```python
from build123d import *

# Parameters (mm, degrees)
SKETCH1_W           = 30
SKETCH1_H           = 80
BOSS_EXTRUDE1_DEPTH = 5
SKETCH2_W           = 5
SKETCH2_H           = 26.5
SKETCH2_H_2         = 5
SKETCH2_R           = 1.5
CUT_EXTRUDE1_DEPTH  = 5
BOSS_EXTRUDE2_DEPTH = 5
FILLET1_R           = 30
SKETCH5_R           = 6.55
SKETCH5_R_2         = 1.5
CUT_EXTRUDE2_DEPTH  = 5
SKETCH6_W           = 16.25
SKETCH6_H           = 5
SKETCH6_R           = 1.5
CUT_EXTRUDE3_DEPTH  = 10
SKETCH7_W           = 5
SKETCH7_H           = 5.5
SKETCH7_H_2         = 10
SKETCH7_H_3         = 6
SKETCH7_R           = 1.5
CUT_EXTRUDE4_DEPTH  = 10
SKETCH8_W           = 5.078430198
SKETCH8_H           = 27.315407993
SKETCH8_W_2         = 5
SKETCH8_H_2         = 26.5
BOSS_EXTRUDE4_DEPTH = 5


with BuildPart() as part:
    # Sketch1 → Boss-Extrude1 (new body)
    with BuildSketch(Plane.XY):
        with BuildLine():
            Line((133.697419571, 70), (-133.697419571, 70))
            ThreePointArc((-133.697419571, 70), (-148.761211935, 47.280628484), (-160, 22.445626465))
            Line((-160, 22.445626465), (-160, -92.445626465))
            ThreePointArc((-160, -92.445626465), (-134.69865165, -138.712454622), (-96.43650761, -175))
            Line((-96.43650761, -175), (96.43650761, -175))
            ThreePointArc((96.43650761, -175), (134.69865165, -138.712454622), (160, -92.445626465))
            Line((160, -92.445626465), (160, 22.445626465))
            ThreePointArc((160, 22.445626465), (148.761211935, 47.280628484), (133.697419571, 70))
        make_face()
        with Locations((-130, 0)):
            Rectangle(SKETCH1_W, SKETCH1_H, mode=Mode.SUBTRACT)
        with Locations((130, 0)):
            Rectangle(SKETCH1_W, SKETCH1_H, mode=Mode.SUBTRACT)
    extrude(amount=BOSS_EXTRUDE1_DEPTH)

    # Sketch2 → Cut-Extrude1 (cut)
    with BuildSketch(Plane.XY.offset(5)):
        with Locations((-97, 0)):
            Rectangle(SKETCH2_W, SKETCH2_H)
        with Locations((-97, 28.75)):
            Rectangle(SKETCH2_W, SKETCH2_H_2)
        with Locations((-97, -28.75)):
            Rectangle(SKETCH2_W, SKETCH2_H_2)
        with Locations((-97, -19.75)):
            Circle(SKETCH2_R)
        with Locations((-97, 19.75)):
            Circle(SKETCH2_R)
    cut_extrude1 = extrude(amount=-CUT_EXTRUDE1_DEPTH, mode=Mode.SUBTRACT)

    # Mirror1: Cut-Extrude1 across plane
    add(cut_extrude1.mirror(Plane(origin=(0, 0, 0), x_dir=(0, 0, 1), z_dir=(1, 0, 0))), mode=Mode.SUBTRACT)

    # Sketch3 → Boss-Extrude2 (add)
    with BuildSketch(Plane.XY.offset(5)):
        with BuildLine():
            ThreePointArc((-2.08e-07, 70), (-3.490893846, 70.285296133), (-6.889142051, 71.133612942))
            Line((-6.889142051, 71.133612942), (-133.697419571, 92))
            Line((-133.697419571, 92), (-133.697419571, 70))
            Line((-133.697419571, 70), (-2.08e-07, 70))
        make_face()
        with BuildLine():
            ThreePointArc((6.889142051, 71.133612942), (3.49089364, 70.285296099), (-2.08e-07, 70))
            Line((-2.08e-07, 70), (133.697419571, 70))
            Line((133.697419571, 70), (133.697419571, 92))
            Line((133.697419571, 92), (6.889142051, 71.133612942))
        make_face()
    extrude(amount=-BOSS_EXTRUDE2_DEPTH)

    # Fillet1
    # the kernel refuses this fillet: 30 mm, written as the material it takes off along each edge
    with BuildSketch(Plane(origin=(-6.889142051, 71.133612942, 9.806082425), x_dir=(-0.9867304131972112, 0.16236715083926523, 0), z_dir=(0, 0, -1))) as fillet1_piece_1:
        with BuildLine():
            CenterArc((1.92243297, -30), FILLET1_R, 90, 6.03368508)
            Line((-1.230961232, -0.166191912), (-1.294029116, 0.430484249))
            ThreePointArc((-1.294029116, 0.430484249), (-0.694557768, 0.502617916), (-0.097420291, 0.592038248))
            Line((-0.097420291, 0.592038248), (0, 0.6))
            Line((0, 0.6), (1.92243297, 0.6))
            Line((1.92243297, 0.6), (1.92243297, 0))
        make_face()
    extrude(amount=14.612164849, mode=Mode.SUBTRACT)
    with BuildSketch(Plane(origin=(6.889142051, 71.133612942, 9.806082425), x_dir=(-0.9561345473491755, -0.29292785351582257, 0), z_dir=(0, 0, -1))) as fillet1_piece_2:
        with BuildLine():
            CenterArc((2.108731211, -29.987480741), FILLET1_R, 91.655317917, 6.03368508)
            Line((-1.905148179, -0.257213803), (-1.985425767, 0.337391536))
            Line((-1.985425767, 0.337391536), (-0.080277588, 0.594605339))
            Line((-0.080277588, 0.594605339), (0.017332037, 0.599749615))
            ThreePointArc((0.017332037, 0.599749615), (0.621064672, 0.591027865), (1.224797306, 0.599749615))
            Line((1.224797306, 0.599749615), (1.242129344, 0))
        make_face()
    extrude(amount=14.612164849, mode=Mode.SUBTRACT)
    with BuildSketch(Plane(origin=(133.697419571, 92, 86.008444254), x_dir=(-0.9867304131972118, -0.16236715083926206, 0), z_dir=(0, 0, -1))) as fillet1_piece_3:
        with BuildLine():
            CenterArc((32.403377702, -30), FILLET1_R, 90, 73.954674896)
            Line((3.572077318, -21.70806909), (2.995451311, -21.542230472))
            ThreePointArc((2.995451311, -21.542230472), (1.194000411, -10.951454836), (-0.592038248, -0.097420291))
            Line((-0.592038248, -0.097420291), (0, 0.6))
            Line((0, 0.6), (32.403377702, 0.6))
            Line((32.403377702, 0.6), (32.403377702, 0))
        make_face()
    extrude(amount=167.016888509, mode=Mode.SUBTRACT)
    with BuildSketch(Plane(origin=(-133.697419571, 92, 86.008444254), x_dir=(0, -1, 0), z_dir=(0, 0, -1))) as fillet1_piece_4:
        with BuildLine():
            CenterArc((34.863156511, -27.102383743), FILLET1_R, 115.389646017, 73.954674896)
            Line((5.261244115, -31.973398269), (4.669205867, -32.070818559))
            Line((4.669205867, -32.070818559), (-0.592038248, -0.097420291))
            Line((-0.592038248, -0.097420291), (0, 0.6))
            ThreePointArc((0, 0.6), (11, 0.6), (21.74273687, 0.542047675))
            Line((21.74273687, 0.542047675), (22, 0))
        make_face()
    extrude(amount=167.016888509, mode=Mode.SUBTRACT)

    # Sketch5 → Cut-Extrude2 (cut)
    with BuildSketch(Plane.XY.offset(5)):
        with Locations((0, -145)):
            Circle(SKETCH5_R)
        with Locations((15, -145)):
            Circle(SKETCH5_R_2)
        with Locations((-15, -145)):
            Circle(SKETCH5_R_2)
    extrude(amount=-CUT_EXTRUDE2_DEPTH, mode=Mode.SUBTRACT)

    # Sketch6 → Cut-Extrude3 (cut)
    with BuildSketch(Plane.XY.offset(5)):
        with Locations((-91.875, -160)):
            Rectangle(SKETCH6_W, SKETCH6_H)
        with Locations((-57.625, -160)):
            Rectangle(SKETCH6_W, SKETCH6_H)
        with Locations((-19.625, -160)):
            Rectangle(SKETCH6_W, SKETCH6_H)
        with Locations((19.625, -160)):
            Rectangle(SKETCH6_W, SKETCH6_H)
        with Locations((57.625, -160)):
            Rectangle(SKETCH6_W, SKETCH6_H)
        with Locations((91.875, -160)):
            Rectangle(SKETCH6_W, SKETCH6_H)
        with Locations((0, -160)):
            Circle(SKETCH6_R)
        with Locations((-74.75, -160)):
            Circle(SKETCH6_R)
        with Locations((74.75, -160)):
            Circle(SKETCH6_R)
    extrude(amount=-CUT_EXTRUDE3_DEPTH, mode=Mode.SUBTRACT)

    # Sketch7 → Cut-Extrude4 (cut)
    with BuildSketch(Plane.XY.offset(5)):
        with Locations((-37.5, 69.75)):
            Rectangle(SKETCH7_W, SKETCH7_H)
        with Locations((-37.5, 51)):
            Rectangle(SKETCH7_W, SKETCH7_H_2)
        with Locations((-72.5, 60)):
            Rectangle(SKETCH7_W, SKETCH7_H_2)
        with Locations((-72.5, 77)):
            Rectangle(SKETCH7_W, SKETCH7_H_3)
        with Locations((-72.5, 43)):
            Rectangle(SKETCH7_W, SKETCH7_H_3)
        with Locations((-37.5, 62.5)):
            Circle(SKETCH7_R)
        with Locations((-72.5, 70.25)):
            Circle(SKETCH7_R)
        with Locations((-72.5, 49.75)):
            Circle(SKETCH7_R)
    cut_extrude4 = extrude(amount=-CUT_EXTRUDE4_DEPTH, mode=Mode.SUBTRACT)

    # Mirror2: Cut-Extrude4 across plane
    add(cut_extrude4.mirror(Plane(origin=(0, 0, 0), x_dir=(0, 0, 1), z_dir=(1, 0, 0))), mode=Mode.SUBTRACT)

    # Sketch8 → Boss-Extrude4 (add)
    with BuildSketch(Plane.XY.offset(5)):
        with Locations((-37.539215099, 59.657703997)):
            Rectangle(SKETCH8_W, SKETCH8_H)
        with Locations((37.5, 59.25)):
            Rectangle(SKETCH8_W_2, SKETCH8_H_2)
    extrude(amount=-BOSS_EXTRUDE4_DEPTH)


solid = part.part
```
Could you check a few things on this model? Use its own coordinates, in mm. A direction names the side the tool comes from. Round coordinates to 2 decimals unless told otherwise and drop trailing zeros. Write each loop counter-clockwise with the first axis right and the second up, starting at its lowest first coordinate (ties: lowest second). Pieces come first, ordered by that corner, then holes. Notation, with made-up numbers: M 47,30 L 100,30 A19 ccw 100,41 Z; hole C -17.5,-26 d6. An arc over 180 degrees is marked long. Answer in a Markdown table with one row per item. Add a question column.
Q1. Imagine slicing it at A-A (x = -121). Please give me the cut outline in (y, z), then the cut area to 3 significant figures.
Q2. Imagine slicing it at B-B (z = 2.55). Give the number of separate pieces and of enclosed holes in the cut face, then the cut area to 3 significant figures.
Q3. If we mould it in two halves opening along Y, with no side actions, what happens to faces 1 (the cylindrical face through (-148.58, 47.61, 2.46)), 2 (the flat face through (-2, -42, 5)), 3 (the cylindrical face through (3.02, -150.81, 2.54))? For each: +Y half, -Y half, draft (parallel to the pull), parting line (faces both ways), or undercut.
Q4. Will these pins go through, and if not, where does the flat tip stop? pin 1 Ø1.5 at (x, z) = (96.5, 2.5) entering from +Y; pin 2 Ø2.5 at (y, z) = (58, 3.5) entering from +X; pin 3 Ø2 at (y, z) = (-130, 1) entering from +X.
Q5. On a 3-axis mill with a long thin cutter (end or side, diameter ignored), from which of +Z, -Z, +X, -X, +Y, -Y can I reach the whole of each face in a straight line? I mean faces 4 (the flat face through (-54.604, 78.985, 2.535)), 5 (the cylindrical face through (148.946, 46.946, 2.465)). Say none if no direction works.
Q6. Imagine slicing it at C-C (x = 35). Please give me the cut outline in (y, z).
Q7. If I drill on line 1 (X direction, y = -26.5, z = 1.7); line 2 (Y direction, x = -72.5, z = 3.9); line 3 (X direction, y = -19, z = 4.55), over which ranges is the centre line in solid material (lowest first)? Write a range as from..to.
Values:
| question | item | result |
|---|---|---|
| 1 | outline | M -154.41,0 L -40,0 L -40,5 L -154.41,5 Z; M 40,0 L 83.45,0 L 83.45,5 L 40,5 Z |
| 1 | area | 789 mm^2 |
| 2 | separate pieces | 1 |
| 2 | enclosed holes | 34 |
| 2 | area | 69,600 mm^2 |
| 3 | face 1 | +Y half |
| 3 | face 2 | draft |
| 3 | face 3 | undercut |
| 4 | pin 1 | y = 86 |
| 4 | pin 2 | x = 143.12 |
| 4 | pin 3 | x = 141.65 |
| 5 | face 4 | +Z, -Z, +Y |
| 5 | face 5 | +Z, -Z, +X, +Y |
| 6 | outline | M -175,0 L 75.76,0 L 75.76,5 L -175,5 Z |
| 7 | line 1 | -160..-145, -115..-99.5, -94.5..94.5, 99.5..115, 145..160 |
| 7 | line 2 | -175..40, 46..48.25, 51.25..55, 65..68.75, 71.75..74, 80..81.93 |
| 7 | line 3 | -160..-145, -115..-98.3, -95.7..95.7, 98.3..115, 145..160 |
